from build123d import *

# Parameters (mm, degrees)
SKETCH_1_R          = 6
SKETCH_1_R_2        = 1.5
EXTRUDE_1_DEPTH     = 6
SKETCH_2_R          = 3.75
CUT_EXTRUDE_1_DEPTH = 1
CUT_EXTRUDE_START   = -1
SKETCH_3_R          = 3.75
CUT_EXTRUDE_2_DEPTH = 1
FILLET_1_R          = 0.5


with BuildPart() as part:
    # 草图1 → 凸台-拉伸1 (new body)
    with BuildSketch(Plane.XY):
        Circle(SKETCH_1_R)
        Circle(SKETCH_1_R_2, mode=Mode.SUBTRACT)
    extrude(amount=EXTRUDE_1_DEPTH)

    # 草图2 → 切除-拉伸1 (cut)
    with BuildSketch(Plane.XY.offset(6)):
        Circle(SKETCH_2_R)
    extrude(amount=-CUT_EXTRUDE_1_DEPTH, mode=Mode.SUBTRACT)

    # 草图3 → 切除-拉伸2 (cut)
    with BuildSketch(Plane(origin=(0, 0, 0), x_dir=(-1, 0, 0), z_dir=(0, 0, -1)).offset(CUT_EXTRUDE_START)):
        with Locations(Location((0, 0, 0), (0, 0, 180))):
            Circle(SKETCH_3_R)
    extrude(amount=CUT_EXTRUDE_2_DEPTH, mode=Mode.SUBTRACT)

    # 圆角1
    fillet_1_edges = [part.edges().sort_by_distance(p)[0] for p in [
        (-6, 0, 0),
        (-6, 0, 6),
    ]]
    fillet(fillet_1_edges, radius=FILLET_1_R)


solid = part.part
Here's how the part is built. I have some questions about the finished solid (model axes, mm). A direction names the side the tool comes from. Give positions to 0.01 mm unless a question says otherwise; leave off trailing zeros. Order: outer loops, then holes, each group sorted by start corner. A loop starts at its lowest first (then second) coordinate and runs counter-clockwise, first axis right, second up. Notation, with made-up numbers: M -39,57 L -4,57 A27 cw -4,85 Z; hole C 8.5,-3 d5. An arc over 180 degrees is marked long. Answer as a JSON object with one key per item and string values. Group by question number.
1) We'd pull the mould along Y, two halves only. Please class faces 4 (the cylindrical face through (-6, 0, 3)), 5 (the cylindrical face through (-1.5, 0.07, 2.97)), 6 (the cylindrical face through (2.02, -3.16, 0.51)), 7 (the flat face through (4, -1, 0)): pulls with the +Y half, pulls with the -Y half, needs draft (parallel to the pull), parting line crosses it, or undercut.
2) Suppose I cut it at A-A, the plane x = 0. Write out the boundary of the cut face in (y, z).
3) Please list where these lines run through material, in increasing order: L1, parallel to Y at x = 0, z = 4.1; L2, parallel to Y at x = 0, z = 5.45; L3, parallel to X at y = -3, z = 5.35. Write a range as [from, to].
4) Suppose I cut it at C-C, the plane z = 4.3. Write out the boundary of the cut face in (x, y), plus the area to 3 significant figures.
5) On a 3-axis mill with a long thin cutter (end or side, diameter ignored), from which of +Z, -Z, +X, -X, +Y, -Y can I reach the whole of each face in a straight line? I mean faces 1 (the flat face through (2, 0, 5)), 2 (the flat face through (2, 0, 1)), 3 (the flat face through (4, -1, 6)). Say none if no direction works.
6) I'm going to push flat-ended pins straight in: pin 1 Ø4 at (x, y) = (0, 0) entering from -Z; pin 2 Ø1.5 at (x, z) = (1.5, 5) entering from +Y; pin 3 Ø6 at (x, y) = (1, -2) entering from -Z; pin 4 Ø6 at (x, y) = (0, 0) entering from +Z. Where does each tip first touch, or does it pass through?
Results found:
{
 "1": {"face 4": "parting line crosses it", "face 5": "undercut", "face 6": "undercut", "face 7": "needs draft"},
 "2": {"outline": "M -6,0.5 A0.5 ccw -5.5,0 L -3.75,0 L -3.75,1 L -1.5,1 L -1.5,5 L -3.75,5 L -3.75,6 L -5.5,6 A0.5 ccw -6,5.5 Z; M 1.5,1 L 3.75,1 L 3.75,0 L 5.5,0 A0.5 ccw 6,0.5 L 6,5.5 A0.5 ccw 5.5,6 L 3.75,6 L 3.75,5 L 1.5,5 Z"},
 "3": {"L1": "[-6, -1.5], [1.5, 6]", "L2": "[-6, -3.75], [3.75, 6]", "L3": "[-5.2, -2.25], [2.25, 5.2]"},
 "4": {"outline": "C 0,0 d12; hole C 0,0 d3", "area": "106 mm²"},
 "5": {"face 1": "+Z", "face 2": "-Z", "face 3": "+Z, +X, -X, +Y, -Y"},
 "6": {"pin 1": "z = 1", "pin 2": "y = 5.95", "pin 3": "z = 0", "pin 4": "z = 5"}
}
